```python
from build123d import *

# Parameters (mm, degrees)
BOSS_EXTRUDE1_DEPTH = 1.6
CUT_EXTRUDE1_DEPTH  = 45.950639595
CUT_EXTRUDE2_DEPTH  = 45.950639595
FILLET1_R           = 5
SKETCH4_W           = 8
SKETCH4_H           = 5
CUT_EXTRUDE3_DEPTH  = 45.950639595
FILLET2_R           = 1
FILLET3_R           = 1
SKETCH6_W           = 24
SKETCH6_H           = 4
CUT_EXTRUDE4_DEPTH  = 45.950639595
SKETCH7_R           = 5
CUT_EXTRUDE5_DEPTH  = 45.950639595
FILLET4_R           = 1
CUT_EXTRUDE6_DEPTH  = 45.950639595
CIRPATTERN1_COUNT   = 2
CIRPATTERN1_ANGLE   = 120
FILLET5_R           = 2


with BuildPart() as part:
    # Sketch1 → Boss-Extrude1 (new body)
    with BuildSketch(Plane(origin=(0, 0, 0), x_dir=(1, 0, 0), z_dir=(0, 1, 0))):
        with BuildLine():
            Line((-9, 5), (18, 5))
            ThreePointArc((18, 5), (43, 0), (18, -5))
            Line((18, -5), (-9, -5))
            Line((-9, -5), (-10, -6))
            Line((-10, -6), (-20.189291565, -6))
            ThreePointArc((-20.189291565, -6), (-41.5, 0), (-20.189291565, 6))
            Line((-20.189291565, 6), (-10, 6))
            Line((-10, 6), (-9, 5))
        make_face()
    extrude(amount=BOSS_EXTRUDE1_DEPTH)

    # Sketch2 → Cut-Extrude1 (cut, through all)
    with BuildSketch(Plane(origin=(0, 0, 0), x_dir=(1, 0, 0), z_dir=(0, 1, 0))):
        with BuildLine():
            Line((40, 1.1), (41, 1.1))
            ThreePointArc((41, 1.1), (42.1, 0), (41, -1.1))
            Line((41, -1.1), (40, -1.1))
            ThreePointArc((40, -1.1), (38.9, 0), (40, 1.1))
        make_face()
        with BuildLine():
            Line((25.952627944, -9.210254038), (25.452627944, -10.076279442))
            ThreePointArc((25.452627944, -10.076279442), (23.95, -10.478907386), (23.547372056, -8.976279442))
            Line((23.547372056, -8.976279442), (24.047372056, -8.110254038))
            ThreePointArc((24.047372056, -8.110254038), (25.55, -7.707626094), (25.952627944, -9.210254038))
        make_face()
        with BuildLine():
            Line((24.047372056, 8.110254038), (23.547372056, 8.976279442))
            ThreePointArc((23.547372056, 8.976279442), (23.95, 10.478907386), (25.452627944, 10.076279442))
            Line((25.452627944, 10.076279442), (25.952627944, 9.210254038))
            ThreePointArc((25.952627944, 9.210254038), (25.55, 7.707626094), (24.047372056, 8.110254038))
        make_face()
    extrude(amount=CUT_EXTRUDE1_DEPTH, mode=Mode.SUBTRACT)

    # Sketch3 → Cut-Extrude2 (cut, through all)
    with BuildSketch(Plane(origin=(0, 0, 0), x_dir=(1, 0, 0), z_dir=(0, 1, 0))):
        with BuildLine():
            Line((-25.047372056, -6.37820323), (-24.547372056, -7.244228634))
            ThreePointArc((-24.547372056, -7.244228634), (-24.95, -8.746856578), (-26.452627944, -8.344228634))
            Line((-26.452627944, -8.344228634), (-26.952627944, -7.47820323))
            ThreePointArc((-26.952627944, -7.47820323), (-26.55, -5.975575286), (-25.047372056, -6.37820323))
        make_face()
        with BuildLine():
            Line((-38, -1.1), (-39, -1.1))
            ThreePointArc((-39, -1.1), (-40.1, 0), (-39, 1.1))
            Line((-39, 1.1), (-38, 1.1))
            ThreePointArc((-38, 1.1), (-36.9, 0), (-38, -1.1))
        make_face()
        with BuildLine():
            Line((-26.952627944, 7.47820323), (-26.452627944, 8.344228634))
            ThreePointArc((-26.452627944, 8.344228634), (-24.95, 8.746856578), (-24.547372056, 7.244228634))
            Line((-24.547372056, 7.244228634), (-25.047372056, 6.37820323))
            ThreePointArc((-25.047372056, 6.37820323), (-26.55, 5.975575286), (-26.952627944, 7.47820323))
        make_face()
    extrude(amount=CUT_EXTRUDE2_DEPTH, mode=Mode.SUBTRACT)

    # Fillet1
    fillet1_edges = [part.edges().sort_by_distance(p)[0] for p in [
        (18, 0.8, 5),
        (-20.189291565, 0.8, 6),
        (-20.189291565, 0.8, -6),
        (18, 0.8, -5),
    ]]
    fillet(fillet1_edges, radius=FILLET1_R)

    # Sketch4 → Cut-Extrude3 (cut, through all)
    with BuildSketch(Plane(origin=(0, 0, 0), x_dir=(1, 0, 0), z_dir=(0, 1, 0))):
        with Locations((-16, 0)):
            Rectangle(SKETCH4_W, SKETCH4_H)
    extrude(amount=CUT_EXTRUDE3_DEPTH, mode=Mode.SUBTRACT)

    # Fillet2
    fillet2_edges = [part.edges().sort_by_distance(p)[0] for p in [
        (-20, 0.8, -2.5),
        (-20, 0.8, 2.5),
        (-12, 0.8, 2.5),
        (-12, 0.8, -2.5),
    ]]
    fillet(fillet2_edges, radius=FILLET2_R)

    # Fillet3
    fillet3_edges = [part.edges().sort_by_distance(p)[0] for p in [
        (-9, 0.8, 5),
        (-10, 0.8, 6),
        (-10, 0.8, -6),
        (-9, 0.8, -5),
    ]]
    fillet(fillet3_edges, radius=FILLET3_R)

    # Sketch6 → Cut-Extrude4 (cut, through all)
    with BuildSketch(Plane(origin=(0, 1.6, 0), x_dir=(1, 0, 0), z_dir=(0, 1, 0))):
        with Locations((9, 0)):
            Rectangle(SKETCH6_W, SKETCH6_H)
    extrude(amount=-CUT_EXTRUDE4_DEPTH, mode=Mode.SUBTRACT)

    # Sketch7 → Cut-Extrude5 (cut, through all)
    with BuildSketch(Plane(origin=(0, 1.6, 0), x_dir=(1, 0, 0), z_dir=(0, 1, 0))):
        with Locations(Location((-30, 0, 0), (0, 0, 270))):
            Circle(SKETCH7_R)
    extrude(amount=-CUT_EXTRUDE5_DEPTH, mode=Mode.SUBTRACT)

    # Fillet4
    fillet4_edges = [part.edges().sort_by_distance(p)[0] for p in [
        (-3, 0.8, 2),
        (-3, 0.8, -2),
        (21, 0.8, -2),
        (21, 0.8, 2),
    ]]
    fillet(fillet4_edges, radius=FILLET4_R)

    # Sketch8 → Cut-Extrude6 (cut, through all)
    with BuildSketch(Plane(origin=(0, 1.6, 0), x_dir=(1, 0, 0), z_dir=(0, 1, 0))):
        with BuildLine():
            Line((27.279443177, 12.712142643), (29.432972741, 8.982120022))
            ThreePointArc((29.432972741, 8.982120022), (34.5, 7.794228634), (38.062257748, 4))
            Line((38.062257748, 4), (42.369316877, 4))
            ThreePointArc((42.369316877, 4), (36.5, 11.258330249), (27.279443177, 12.712142643))
        make_face()
    cut_extrude6 = extrude(amount=-CUT_EXTRUDE6_DEPTH, mode=Mode.SUBTRACT)

    # CirPattern1: Cut-Extrude6 ×2 about axis
    cirpattern1_axis = Axis((30, 0, 0), (0, -1, 0))
    for i in range(1, CIRPATTERN1_COUNT):
        add(cut_extrude6.rotate(cirpattern1_axis, i * CIRPATTERN1_ANGLE / (CIRPATTERN1_COUNT - 1)), mode=Mode.SUBTRACT)

    # Fillet5
    fillet5_edges = [part.edges().sort_by_distance(p)[0] for p in [
        (27.279443177, 0.8, -12.712142643),
        (42.369316877, 0.8, -4),
        (38.062257748, 0.8, -4),
        (29.432972741, 0.8, -8.982120022),
        (42.369316877, 0.8, 4),
        (27.279443177, 0.8, 12.712142643),
        (29.432972741, 0.8, 8.982120022),
        (38.062257748, 0.8, 4),
    ]]
    fillet(fillet5_edges, radius=FILLET5_R)


solid = part.part
```
Work out the finished part from the listing and answer in its coordinate system (mm). A direction names the side the tool comes from. Round coordinates to 2 decimals unless told otherwise and drop trailing zeros. Loops run counter-clockwise (first coordinate to the right, second up) from the corner with the lowest first, then second, coordinate; pieces in that order, holes last. Notation, with made-up numbers: (88.25, 13.25) -> (95.25, 13.25) arc R31 cw to (95.25, 38.25) -> close; hole circle Ø9 at (-8, 66.5). An arc over 180 degrees is marked (long way). Write each question's results on one line, items separated by ' | '. Start each with the question number.
1. A tool of negligible diameter and unlimited length cuts with its end or side. For faces 5 (the face through (40, 1, -4)), 6 (the face through (-16, 1, 2.5)), 7 (the face through (17.421, 0.811, 5.607)), from which of +Z, -Z, +X, -X, +Y, -Y can it reach the whole face along a straight path? Write none if from no direction.
2. Section C-C (y = 0.25) is taken. State how many separate pieces and enclosed holes the cut face has, plus the area to 3 significant figures.
3. Section A-A (x = -30) is taken. Determine the outline of the cut face in (y, z).
4. Given pin 1 Ø0.8 at (x, y) = (9, 1) entering from +Z; pin 2 Ø0.5 at (x, y) = (40, 0.5) entering from -Z; pin 3 Ø0.8 at (x, y) = (-13, 1) entering from +Z; pin 4 Ø3 at (x, z) = (-25, 7.5) entering from +Y, each flat-ended and moving along its own axis, determine where each tip first touches the part or whether it passes through.
5. Find the intervals of material crossed by probe 1 along X at (y, z) = (0.9, 0); probe 2 along X at (y, z) = (1.5, -8); probe 3 along X at (y, z) = (1.5, 7.25), in increasing order. Write a range as from..to.
6. Section B-B (z = 0) is taken. Determine the outline of the cut face in (x, y), plus the area to 3 significant figures.
7. For a pull along Z with two mould halves and no side action, classify faces 1 (the face through (38.25, 0.79, 4.25)), 2 (the face through (21.971, 0.789, -10.224)), 3 (the face through (-12, 1, 0)), 4 (the face through (9, 1, -2)) as +Z half, -Z half, draft (parallel to the pull), parting line (faces both ways), or undercut.
Evaluation:
1) face 5: -Z, +X, +Y, -Y | face 6: +Y, -Y | face 7: +Z, +Y, -Y
2) separate pieces: 1 | enclosed holes: 9 | area: 965 mm2
3) outline: (0, -11.5) -> (1.6, -11.5) -> (1.6, -5) -> (0, -5) -> close; (0, 5) -> (1.6, 5) -> (1.6, 11.5) -> (0, 11.5) -> close
4) pin 1: stops at z = 5 | pin 2: stops at z = -4 | pin 3: stops at z = 6 | pin 4: stops at y = 1.6
5) probe 1: x = -41.5..-40.1, -36.9..-35, -25..-20, -12..-3, 21..38.9, 42.1..43 | probe 2: x = -38.26..-26.65, -24.42..-21.74, 19.75..24.12, 25.88..34.12 | probe 3: x = -38.93..-27.05, -24.54..-21.01, 19.21..35.33
6) outline: (-41.5, 0) -> (-40.1, 0) -> (-40.1, 1.6) -> (-41.5, 1.6) -> close; (-36.9, 0) -> (-35, 0) -> (-35, 1.6) -> (-36.9, 1.6) -> close; (-25, 0) -> (-20, 0) -> (-20, 1.6) -> (-25, 1.6) -> close; (-12, 0) -> (-3, 0) -> (-3, 1.6) -> (-12, 1.6) -> close; (21, 0) -> (38.9, 0) -> (38.9, 1.6) -> (21, 1.6) -> close; (42.1, 0) -> (43, 0) -> (43, 1.6) -> (42.1, 1.6) -> close | area: 57.8 mm2
7) face 1: +Z half | face 2: -Z half | face 3: undercut | face 4: undercut
